Check sheet for the modelled part. Datum: model origin and axes. Units: mm. Face numbers are marked on the shaded views. Coordinates: 2 decimals unless noted, no trailing zeros. Loops run counter-clockwise (first coordinate to the right, second up) from the corner with the lowest first, then second, coordinate; pieces in that order, holes last. Notation, with made-up numbers: (53, -4.75) -> (60, -4.75) arc R20 cw to (60, 19.25) -> close; hole circle Ø11 at (50.5, -13.75). An arc over 180 degrees is marked (long way). Use CSV: the item, a comma, the result in double quotes. Start each with the question number.
1. Sectioned sample at B-B, the plane z = 3.1. Record the cut outline in (x, y).
2. Gauge pin test, flat ends, axial feed: pin 1 (3 mm diameter, centred on x = -11.5, z = 5, fed in from -Y); pin 2 (2 mm diameter, centred on y = 12, z = 2, fed in from -X). Record the tip position at first contact, or that the pin passes through.
3. Sectioned sample at D-D, the plane y = -12. Record the cut outline in (x, z).
4. Release check for a two-part mould opening along X. For the marked faces 1, 2 and 3 record: pulls with the +X half, pulls with the -X half, needs draft (parallel to the pull), parting line crosses it, or undercut.
5. Sectioned sample at C-C, the plane y = 0. Record the cut outline in (x, z), and give its area (3 significant figures).
6. Thickness scan on L1, parallel to Y at x = 0, z = 2.75; L2, parallel to X at y = -1, z = 3.1; L3, parallel to Y at x = -6, z = 0.7. Record the ranges inside material, lowest first.
7. Sectioned sample at A-A, the plane x = 0. Record the cut outline in (y, z), and give its area (3 significant figures).
```python
from build123d import *

# Parameters (mm, degrees)
SKETCH1_R                = 17.229166667
SKETCH1_R_2              = 3
BOSS_EXTRUDE1_DEPTH      = 5.8
SKETCH2_R                = 0.79375
CUT_EXTRUDE1_DEPTH       = 26.046524071
M3_CLEARANCE_HOLE1_D     = 3.2
M3_CLEARANCE_HOLE1_DEPTH = 12.7
M3_CLEARANCE_HOLE1_TIP   = 0.96137699


with BuildPart() as part:
    # Sketch1 → Boss-Extrude1 (new body)
    with BuildSketch(Plane.XY):
        Circle(SKETCH1_R)
        Circle(SKETCH1_R_2, mode=Mode.SUBTRACT)
    extrude(amount=BOSS_EXTRUDE1_DEPTH)

    # Sketch2 → Cut-Extrude1 (cut, through all)
    with BuildSketch(Plane.XY.offset(5.8)):
        with Locations((0, 12)):
            Circle(SKETCH2_R)
        with Locations((12, 0)):
            Circle(SKETCH2_R)
        with Locations((0, -12)):
            Circle(SKETCH2_R)
        with Locations((-12, 0)):
            Circle(SKETCH2_R)
    extrude(amount=-CUT_EXTRUDE1_DEPTH, mode=Mode.SUBTRACT)

    # M3 Clearance Hole1
    with Locations(Plane.XY.offset(5.8)):
        with Locations((-6, 0), (6, 0)):
            Hole(M3_CLEARANCE_HOLE1_D / 2, depth=M3_CLEARANCE_HOLE1_DEPTH)
            with Locations((0, 0, -(M3_CLEARANCE_HOLE1_DEPTH + M3_CLEARANCE_HOLE1_TIP / 2))):  # 118° drill point
                Cone(0, M3_CLEARANCE_HOLE1_D / 2, M3_CLEARANCE_HOLE1_TIP, mode=Mode.SUBTRACT)


solid = part.part
```
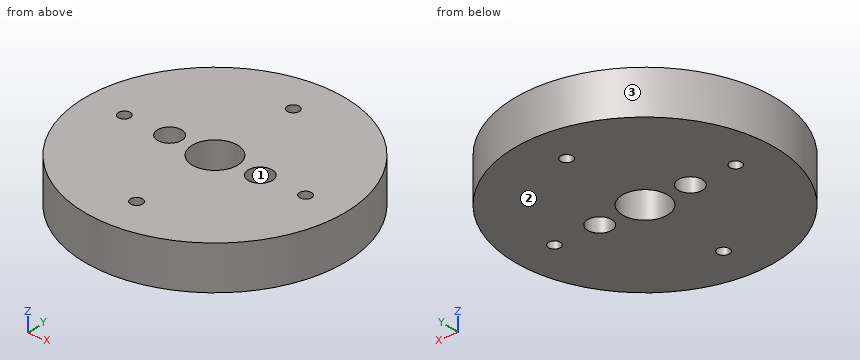
Completed:
1,outline,"circle Ø34.46 at (0, 0); hole circle Ø1.59 at (-12, 0); hole circle Ø3.2 at (-6, 0); hole circle Ø6 at (0, 0); hole circle Ø1.59 at (0, -12); hole circle Ø1.59 at (0, 12); hole circle Ø3.2 at (6, 0); hole circle Ø1.59 at (12, 0)"
2,pin 1,"y = -14.03"
2,pin 2,"x = -13.26"
3,outline,"(-12.36, 0) -> (-0.79, 0) -> (-0.79, 5.8) -> (-12.36, 5.8) -> close; (0.79, 0) -> (12.36, 0) -> (12.36, 5.8) -> (0.79, 5.8) -> close"
4,face 1,"undercut"
4,face 2,"needs draft"
4,face 3,"parting line crosses it"
5,outline,"(-17.23, 0) -> (-12.79, 0) -> (-12.79, 5.8) -> (-17.23, 5.8) -> close; (-11.21, 0) -> (-7.6, 0) -> (-7.6, 5.8) -> (-11.21, 5.8) -> close; (-4.4, 0) -> (-3, 0) -> (-3, 5.8) -> (-4.4, 5.8) -> close; (3, 0) -> (4.4, 0) -> (4.4, 5.8) -> (3, 5.8) -> close; (7.6, 0) -> (11.21, 0) -> (11.21, 5.8) -> (7.6, 5.8) -> close; (12.79, 0) -> (17.23, 0) -> (17.23, 5.8) -> (12.79, 5.8) -> close"
5,area,"110 mm²"
6,L1,"-17.23 to -12.79, -11.21 to -3, 3 to 11.21, 12.79 to 17.23"
6,L2,"-17.2 to -7.25, -4.75 to -2.83, 2.83 to 4.75, 7.25 to 17.2"
6,L3,"-16.15 to -1.6, 1.6 to 16.15"
7,outline,"(-17.23, 0) -> (-12.79, 0) -> (-12.79, 5.8) -> (-17.23, 5.8) -> close; (-11.21, 0) -> (-3, 0) -> (-3, 5.8) -> (-11.21, 5.8) -> close; (3, 0) -> (11.21, 0) -> (11.21, 5.8) -> (3, 5.8) -> close; (12.79, 0) -> (17.23, 0) -> (17.23, 5.8) -> (12.79, 5.8) -> close"
7,area,"147 mm²"
